Autodesk Fusion 360 part; units mm, degrees
sketch "Sketch1" plane through (0, 0, 0) normal (0, 0, 1) x (1, 0, 0)
  line L0 (-6.35, 9.525) -> (6.35, 9.525)
  line L1 (6.35, 9.525) -> (6.35, -9.525)
  line L2 (6.35, -9.525) -> (-6.35, -9.525)
  line L3 (-6.35, -9.525) -> (-6.35, 9.525)
  line L4 (0, 0) -> (0, 3.175) construction
  line L5 (0, 3.175) -> (0, 6.35) construction
  line L6 (0, 0) -> (0, -3.175) construction
  line L7 (0, -3.175) -> (0, -6.35) construction
  circle A0 centre (0, 6.35) radius 1.5875
  circle A1 centre (0, 3.175) radius 1.5875
  circle A2 centre (0, 0) radius 1.5875
  circle A3 centre (0, -3.175) radius 1.5875
  circle A4 centre (0, -6.35) radius 1.5875
  arc A5 (6.35, 3.175) -> (6.35, -3.175) centre (6.35, 0) ccw
  dimension "d3" = 12.7
  dimension "d4" = 19.05
  dimension "d5" = 3.175
  dimension "d6" = 3.175
  dimension "d7" = 3.175
  dimension "d8" = 3.175
  dimension "d9" = 3.175
  dimension "d10" = 3.175
  dimension "d11" = 3.175
  dimension "d12" = 3.175
  dimension "d13" = 3.175
  dimension "d21" = 6.35
extrude "Extrude1" add sketch "Sketch1" along normal blind 6.35 contours L0 L1 L2 L3 A5
sketch "Sketch2" plane through (0, 0, 6.35) normal (0, 0, 1) x (-1, 0, 0)
  circle A0 centre (0, 6.35) radius 1.5875
  circle A1 centre (0, -6.35) radius 1.5875
  line L0 (6.35, 9.525) -> (-6.35, 9.525)
  line L1 (-6.35, -3.175) -> (-6.35, -9.525)
  line L2 (-6.35, -9.525) -> (6.35, -9.525)
  line L3 (6.35, -9.525) -> (6.35, 9.525)
  arc A2 (1.905, 6.35) -> (-1.905, 6.35) centre (0, 6.35) ccw
  arc A3 (-1.905, -6.35) -> (1.905, -6.35) centre (0, -6.35) ccw
  circle A4 centre (0, -3.175) radius 1.5875
  arc A5 (0, -1.5875) -> (0, 1.5875) centre (0, 0) ccw
  arc A6 (0, 1.5875) -> (0, 4.7625) centre (0, 3.175) ccw
  arc A7 (0, -1.5875) -> (0, -4.7625) centre (0, -3.175) ccw
  arc A8 (0, 1.5875) -> (0, -1.5875) centre (0, 0) ccw
  arc A9 (0, 4.7625) -> (0, 1.5875) centre (0, 3.175) ccw
  line L4 (-6.35, 9.525) -> (-6.35, 3.175)
  arc A10 (-6.35, -3.175) -> (-6.35, 3.175) centre (-6.35, 0) ccw
  dimension "d17" = 3.81
  dimension "d18" = 3.81
sketch "Sketch3" plane through (0, 0, 6.35) normal (0, 0, 1) x (-1, 0, 0)
  circle A0 centre (0, 6.35) radius 1.5875
  arc A1 (0, 1.5875) -> (0, 4.7625) centre (0, 3.175) ccw
  arc A2 (0, -1.5875) -> (0, 1.5875) centre (0, 0) ccw
  arc A3 (0, -4.7625) -> (0, -1.5875) centre (0, -3.175) ccw
  circle A4 centre (0, -6.35) radius 1.5875
  arc A5 (0, -1.5875) -> (0, -4.7625) centre (0, -3.175) ccw
  arc A6 (0, 1.5875) -> (0, -1.5875) centre (0, 0) ccw
  arc A7 (0, 4.7625) -> (0, 1.5875) centre (0, 3.175) ccw
  line L0 (-6.35, -3.175) -> (-6.35, -9.525)
  line L1 (-6.35, -9.525) -> (6.35, -9.525)
  line L2 (6.35, -9.525) -> (6.35, 9.525)
  line L3 (6.35, 9.525) -> (-6.35, 9.525)
  line L4 (-6.35, 9.525) -> (-6.35, 3.175)
  arc A8 (-6.35, -3.175) -> (-6.35, 3.175) centre (-6.35, 0) ccw
sketch "Sketch4" plane through (-6.35, 0, 0) normal (-1, 0, 0) x (0, -1, 0)
  line L0 (-9.525, 0) -> (9.525, 0)
  line L1 (9.525, 0) -> (9.525, 6.35)
  line L2 (9.525, 6.35) -> (-9.525, 6.35)
  line L3 (-9.525, 6.35) -> (-9.525, 0)
  line L4 (0, 0) -> (0, 3.175) construction
  circle A0 centre (0, 3.175) radius 1.905
  dimension "d22" = 3.175
  dimension "d23" = 3.81
extrude "Extrude3" cut sketch "Sketch4" against normal blind 3.81 contours A0
thread "Thread1" thread offset 0 thread length 10.0076
equation "d9 = ( 1 / 8 ) * 1 in"
equation "d10 = ( 1 / 8 ) * 1 in"
equation "d11 = ( 1 / 8 ) * 1 in"
equation "d13 = ( 1 / 8 ) * 1 in"
equation "d21 = ( 1 / 4 ) * 1 in"
equation "d22 = ( 1 / 8 ) * 1 in"
Geometry: final body of the model. Coordinates: model frame, mm. A direction names the side the tool comes from. Coordinates: 2 decimals unless noted, no trailing zeros. Order: outer loops, then holes, each group sorted by start corner. A loop starts at its lowest first (then second) coordinate and runs counter-clockwise, first axis right, second up. Notation, with made-up numbers: M 23,-39 L 67,-39 A17 cw 67,-35 Z; hole C 64,-9.75 d5. An arc over 180 degrees is marked long. Answer in a Markdown table with one row per item. Add a question column.
Q1. Reachability of faces 4 (the flat face through (-6.35, -0.13, 5.25)), 5 (the cylindrical face through (-4.472, 0.248, 5.064)), 6 (the cylindrical face through (-1.587, -3.21, 3.131)) from +Z, -Z, +X, -X, +Y, -Y: full face, straight path, thin tool, end or side. Return the list, or none.
Q2. Contact query for flat-ended pins moving along their axis: P1, Ø5, axis at x = 0.5, y = -2, coming from the +Z side; P2, Ø1.9, axis at x = 0, y = 6.35, coming from the +Z side. Output: stop coordinate, or through.
Q3. Section query D-D on y = -4. Return the cut outline in (x, z).
Q4. Mould query, pull axis Y, two halves, no side actions, for faces 1 (the flat face through (0, 9.525, 3)), 2 (the cylindrical face through (1.587, 3.21, 3.131)), 3 (the flat face through (-2, 2, 0)). Classes: released by +Y, released by -Y, zero draft, split by the parting line, or undercut.
Q5. Line query: L1, parallel to X at y = 6.35, z = 4; L2, parallel to Y at x = 0.5, z = 4.5 (3 decimals); L3, parallel to Y at x = 1, z = 4.5 (3 decimals). Output: solid intervals per line, ascending.
Q6. Section query B-B on x = -4.25. Return the cut outline in (y, z) (3 decimals).
Completed:
| question | item | result |
|---|---|---|
| 1 | face 4 | +Z, -Z, -X, +Y, -Y |
| 1 | face 5 | -X |
| 1 | face 6 | +Z, -Z |
| 2 | P1 | stops at z = 6.35 |
| 2 | P2 | passes through |
| 3 | outline | M -6.35,0 L -1.36,0 L -1.36,6.35 L -6.35,6.35 Z; M 1.36,0 L 6.35,0 L 6.35,6.35 L 1.36,6.35 Z |
| 4 | face 1 | released by +Y |
| 4 | face 2 | undercut |
| 4 | face 3 | zero draft |
| 5 | L1 | x = -6.35 to -1.59, 1.59 to 6.35 |
| 5 | L2 | y = -9.525 to -7.857, -4.843 to -4.682, -1.668 to -1.507, 1.507 to 1.668, 4.682 to 4.843, 7.857 to 9.525 |
| 5 | L3 | y = -9.525 to -7.583, -5.117 to -4.408, -1.942 to -1.233, 1.233 to 1.942, 4.408 to 5.117, 7.583 to 9.525 |
| 6 | outline | M -9.525,0 L 9.525,0 L 9.525,6.35 L -9.525,6.35 Z; hole C 0,3.175 d3.81 |
